```python
from build123d import *

# Parameters (mm, degrees)
SKETCH1_W           = 100
SKETCH1_H           = 100
BOSS_EXTRUDE1_DEPTH = 6.35
SKETCH2_W           = 12.7
SKETCH2_H           = 6.35
BOSS_EXTRUDE2_DEPTH = 6.35
CIRPATTERN1_COUNT   = 3
CIRPATTERN1_ANGLE   = 180
SKETCH4_W           = 12.7
SKETCH4_H           = 6.35
BOSS_EXTRUDE3_DEPTH = 59.05
SKETCH5_W           = 40
SKETCH5_H           = 40
CUT_EXTRUDE1_DEPTH  = 7.35
SKETCH6_W           = 6.35
SKETCH6_H           = 12.7
CUT_EXTRUDE2_DEPTH  = 7.35


with BuildPart() as part:
    # Sketch1 → Boss-Extrude1 (new body)
    with BuildSketch(Plane(origin=(0, 0, 0), x_dir=(1, 0, 0), z_dir=(0, 1, 0))):
        Rectangle(SKETCH1_W, SKETCH1_H)
    extrude(amount=BOSS_EXTRUDE1_DEPTH)

    # Sketch2 → Boss-Extrude2 (add)
    with BuildSketch(Plane.ZY.offset(50)):
        with Locations((0, 3.175)):
            Rectangle(SKETCH2_W, SKETCH2_H)
    boss_extrude2 = extrude(amount=BOSS_EXTRUDE2_DEPTH)

    # CirPattern1: Boss-Extrude2 ×3 about axis
    cirpattern1_axis = Axis((0, 0, 0), (0, 1, 0))
    for i in range(1, CIRPATTERN1_COUNT):
        add(boss_extrude2.rotate(cirpattern1_axis, i * CIRPATTERN1_ANGLE / (CIRPATTERN1_COUNT - 1)))

    # Sketch4 → Boss-Extrude3 (add)
    with BuildSketch(Plane.XY.offset(50)):
        with Locations((-43.65, 3.175)):
            Rectangle(SKETCH4_W, SKETCH4_H)
    boss_extrude3 = extrude(amount=BOSS_EXTRUDE3_DEPTH)

    # Mirror1: Boss-Extrude3 across plane
    add(boss_extrude3.mirror(Plane(origin=(0, 0, 0), x_dir=(0, 0, 1), z_dir=(1, 0, 0))))

    # Sketch5 → Cut-Extrude1 (cut, through all)
    with BuildSketch(Plane(origin=(0, 6.35, 0), x_dir=(1, 0, 0), z_dir=(0, 1, 0))):
        with Locations((0, 23.65)):
            Rectangle(SKETCH5_W, SKETCH5_H)
    extrude(amount=-CUT_EXTRUDE1_DEPTH, mode=Mode.SUBTRACT)

    # Sketch6 → Cut-Extrude2 (cut, through all)
    with BuildSketch(Plane(origin=(0, 6.35, 0), x_dir=(1, 0, 0), z_dir=(0, 1, 0))):
        with Locations((-16.825, -2.7)):
            Rectangle(SKETCH6_W, SKETCH6_H)
    cut_extrude2 = extrude(amount=-CUT_EXTRUDE2_DEPTH, mode=Mode.SUBTRACT)

    # Mirror2: Cut-Extrude2 across plane
    add(cut_extrude2.mirror(Plane(origin=(0, 0, 0), x_dir=(0, 0, 1), z_dir=(1, 0, 0))), mode=Mode.SUBTRACT)


solid = part.part
```
For this review, take the finished solid that the model builds, in its own axes (mm). A direction names the side the tool comes from. Coordinates: 2 decimals unless noted, no trailing zeros. Order: outer loops, then holes, each group sorted by start corner. A loop starts at its lowest first (then second) coordinate and runs counter-clockwise, first axis right, second up. Notation, with made-up numbers: (33, 24) - (59, 24) arc R17 ccw to (59, 31) - close; hole circle Ø7 at (29.5, 72). An arc over 180 degrees is marked (long way). Answer as a JSON object with one key per item and string values. Group by question number.
1. For faces 4 (the flat face through (22, 3, 50)), 5 (the flat face through (53, 3, -6.35)), 6 (the flat face through (13.65, 3, 3)), 7 (the flat face through (-12, 6.35, 11)), 8 (the flat face through (-53, 3, -6.35)), list the 3-axis set-ups (+Z, -Z, +X, -X, +Y, -Y) from which the entire face can be reached by the end or side of a thin tool; tool diameter is ignored.
2. Clearance check with flat-ended pins moving along their axes: P1, Ø1.9, axis at y = 1.5, z = 52.5, coming from the +X side; P2, Ø1.9, axis at x = -1, y = 2.5, coming from the +Z side; P3, Ø1.9, axis at x = -17, y = 3, coming from the +Z side. State where each tip first meets the part, or that it passes through.
3. We need section A-A on z = -33. State the section outline as (x, y) points, then the cut area to 3 significant figures.
4. For probe 1 along X at (y, z) = (4, 7.5); probe 2 along X at (y, z) = (0.75, 86); probe 3 along Z at (x, y) = (19, 3), list the stretches that pass through material, from the lowest coordinate up.
5. We need section D-D on z = 4. State the section outline as (x, y) points.
6. The part is to be moulded in two halves that separate along X. For faces 1 (the flat face through (56.35, 3, 0)), 2 (the flat face through (-1, 3, -50)), 3 (the flat face through (-20, 3, -17)), say which applies: pulls with the +X half, pulls with the -X half, needs draft (parallel to the pull), parting line crosses it, or undercut.
7. We need section B-B on x = 4. State the section outline as (y, z) points, then the cut area to 3 significant figures.
8. We need section C-C on y = 2. State the section outline as (x, z) points, then the cut area to 3 significant figures.
Final values:
{
 "1": {"face 4": "+Z, +Y, -Y", "face 5": "-Z, +X, +Y, -Y", "face 6": "+Y, -Y", "face 7": "+Z, -Z, +X, -X, +Y", "face 8": "-Z, -X, +Y, -Y"},
 "2": {"P1": "x = 50", "P2": "z = 56.35", "P3": "z = 50"},
 "3": {"outline": "(-50, 0) - (-20, 0) - (-20, 6.35) - (-50, 6.35) - close; (20, 0) - (50, 0) - (50, 6.35) - (20, 6.35) - close", "area": "381 mm²"},
 "4": {"probe 1": "-50 to -20, -13.65 to 13.65, 20 to 50", "probe 2": "-50 to -37.3, 37.3 to 50", "probe 3": "-50 to -43.65, 9.05 to 50"},
 "5": {"outline": "(-56.35, 0) - (-20, 0) - (-20, 6.35) - (-56.35, 6.35) - close; (-13.65, 0) - (13.65, 0) - (13.65, 6.35) - (-13.65, 6.35) - close; (20, 0) - (56.35, 0) - (56.35, 6.35) - (20, 6.35) - close"},
 "6": {"face 1": "pulls with the +X half", "face 2": "needs draft", "face 3": "undercut"},
 "7": {"outline": "(0, -50) - (6.35, -50) - (6.35, -43.65) - (0, -43.65) - close; (0, -3.65) - (6.35, -3.65) - (6.35, 56.35) - (0, 56.35) - close", "area": "421 mm²"},
 "8": {"outline": "(-56.35, -6.35) - (-50, -6.35) - (-50, -50) - (50, -50) - (50, -6.35) - (56.35, -6.35) - (56.35, 6.35) - (50, 6.35) - (50, 109.05) - (37.3, 109.05) - (37.3, 50) - (6.35, 50) - (6.35, 56.35) - (-6.35, 56.35) - (-6.35, 50) - (-37.3, 50) - (-37.3, 109.05) - (-50, 109.05) - (-50, 6.35) - (-56.35, 6.35) - close; hole (-20, -43.65) - (20, -43.65) - (20, 9.05) - (13.65, 9.05) - (13.65, -3.65) - (-13.65, -3.65) - (-13.65, 9.05) - (-20, 9.05) - close", "area": "9,980 mm²"}
}
